Work out the finished part from the listing and answer in its coordinate system (mm). Face numbers are marked on the shaded views. A direction names the side the tool comes from. Give positions to 0.01 mm unless a question says otherwise; leave off trailing zeros. Loops run counter-clockwise (first coordinate to the right, second up) from the corner with the lowest first, then second, coordinate; pieces in that order, holes last. Notation, with made-up numbers: M 12.25,25.5 L 63.25,25.5 A28 cw 63.25,47.5 Z; hole C -11.5,80.25 d8. An arc over 180 degrees is marked long. Answer as a JSON object with one key per item and string values. Group by question number.
```python
from build123d import *

# Parameters (mm, degrees)
F1_DEPTH = 12.7


with BuildPart() as f1:
    # F0 (on Front) → F1 (new body)
    with BuildSketch(Plane.XZ):
        with BuildLine():
            Line((0, -10.849522), (0, 0))
            Line((0, 0), (-38.862, 0))
            ThreePointArc((-38.862, 0), (-39.825896, 0.399259), (-40.225154, 1.363154))
            Line((-40.225154, 1.363154), (-40.225154, 2.830707))
            Line((-40.225154, 2.830707), (-49.026658, 0))
            Line((-49.026658, 0), (-49.026658, -6.0248))
            ThreePointArc((-49.026658, -6.0248), (-34.110593, -2.19715), (-19.100076, -5.635793))
            ThreePointArc((-19.100076, -5.635793), (-18.549908, -6.13839), (-18.34623, -6.855191))
            Line((-18.34623, -6.855191), (-18.34623, -10.849522))
            Line((-18.34623, -10.849522), (0, -10.849522))
        make_face()
        with BuildLine():
            Line((38.862, 0), (0, 0))
            Line((0, 0), (0, -10.849522))
            Line((0, -10.849522), (18.34623, -10.849522))
            Line((18.34623, -10.849522), (18.34623, -6.855191))
            ThreePointArc((18.34623, -6.855191), (18.549908, -6.13839), (19.100076, -5.635793))
            ThreePointArc((19.100076, -5.635793), (34.110593, -2.19715), (49.026658, -6.0248))
            Line((49.026658, -6.0248), (49.026658, 0))
            Line((49.026658, 0), (40.225154, 2.830707))
            Line((40.225154, 2.830707), (40.225154, 1.363154))
            ThreePointArc((40.225154, 1.363154), (39.825896, 0.399259), (38.862, 0))
        make_face()
    extrude(amount=F1_DEPTH)


solid = f1.part
```
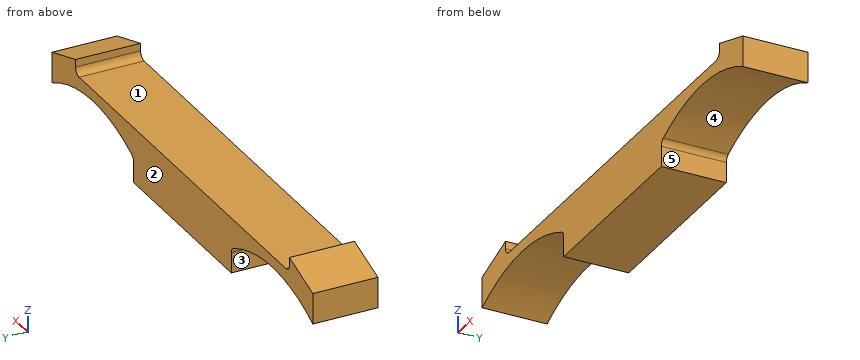
Item 1: A cutting plane is placed at A-A (y = -1.5). Determine the outline of the cut face in (x, z), and give its area (3 significant figures).
Item 2: A cutting plane is placed at B-B (z = -3.25). Determine the outline of the cut face in (x, y), and give its area (3 significant figures).
Item 3: For a pull along X with two mould halves and no side action, classify the marked faces 3, 4 and 5 as pulls with the +X half, pulls with the -X half, needs draft (parallel to the pull), parting line crosses it, or undercut.
Item 4: Given pin 1 Ø2 at (x, z) = (-21, -2) entering from +Y; pin 2 Ø4.5 at (y, z) = (-9, -8.5) entering from +X; pin 3 Ø3 at (y, z) = (-9, -9) entering from -X, each flat-ended and moving along its own axis, determine where each tip first touches the part or whether it passes through.
Item 5: A cutting plane is placed at C-C (x = -6.5). Determine the outline of the cut face in (y, z), and give its area (3 significant figures).
Item 6: A tool of negligible diameter and unlimited length cuts with its end or side. For the marked faces 1 and 2, from which of +Z, -Z, +X, -X, +Y, -Y can it reach the whole face along a straight path? Write none if from no direction.
Item 7: Find the intervals of material crossed by probe 1 along X at (y, z) = (-4.5, -5.25); probe 2 along X at (y, z) = (-10, -4.5); probe 3 along Z at (x, y) = (-9.5, -7.5), in increasing order. Write a range as [from, to].
Item 8: A cutting plane is placed at D-D (z = -7.75). Determine the outline of the cut face in (x, y).
The answers:
{
 "1": {"outline": "M -49.03,-6.02 A32.63 cw -19.1,-5.64 A1.36 cw -18.35,-6.86 L -18.35,-10.85 L 18.35,-10.85 L 18.35,-6.86 A1.36 cw 19.1,-5.64 A32.63 cw 49.03,-6.02 L 49.03,0 L 40.23,2.83 L 40.23,1.36 A1.36 cw 38.86,0 L -38.86,0 A1.36 cw -40.23,1.36 L -40.23,2.83 L -49.03,0 Z", "area": "635 mm^2"},
 "2": {"outline": "M -49.03,-12.7 L -41.92,-12.7 L -41.92,0 L -49.03,0 Z; M -25.45,-12.7 L 25.45,-12.7 L 25.45,0 L -25.45,0 Z; M 41.92,-12.7 L 49.03,-12.7 L 49.03,0 L 41.92,0 Z", "area": "827 mm^2"},
 "3": {"face 3": "pulls with the -X half", "face 4": "undercut", "face 5": "pulls with the +X half"},
 "4": {"pin 1": "stops at y = 0", "pin 2": "stops at x = 18.49", "pin 3": "stops at x = -18.35"},
 "5": {"outline": "M -12.7,-10.85 L 0,-10.85 L 0,0 L -12.7,0 Z", "area": "138 mm^2"},
 "6": {"face 1": "+Z, +Y, -Y", "face 2": "+Z, -Z, +X, -X, +Y"},
 "7": {"probe 1": "x = [-49.03, -47.47], [-19.9, 19.9], [47.47, 49.03]", "probe 2": "x = [-49.03, -45.73], [-21.64, 21.64], [45.73, 49.03]", "probe 3": "z = [-10.85, 0]"},
 "8": {"outline": "M -18.35,-12.7 L 18.35,-12.7 L 18.35,0 L -18.35,0 Z"}
}
